Read the model definition and answer for the solid it produces. Units are mm, in the model's axes. A direction names the side the tool comes from. Round coordinates to 2 decimals unless told otherwise and drop trailing zeros. Order: outer loops, then holes, each group sorted by start corner. A loop starts at its lowest first (then second) coordinate and runs counter-clockwise, first axis right, second up. Notation, with made-up numbers: (28.5, 25) - (63.5, 25) arc R21 ccw to (63.5, 55) - close; hole circle Ø11 at (62.5, 3.5). An arc over 180 degrees is marked (long way). One line per question, with ' | ' between items. Start each with the question number.
1) The part is cut by section D-D, the plane x = -1.5. Give the vertices of the cut face in (y, z), plus the area to 3 significant figures.
2) Flat-ended cylindrical pins translate along their axes: pin 1 (2.5 mm diameter, centred on y = -5, z = 0, fed in from +X); pin 2 (0.5 mm diameter, centred on x = 2, y = -3, fed in from -Z); pin 3 (1.5 mm diameter, centred on y = -4, z = 0, fed in from -X). Find the tip coordinate at first contact, or state that the pin passes through.
3) For faces 1 (the flat face through (4.5, -1, 0)), 2 (the flat face through (-1.25, -4, 1)), 3 (the flat face through (2, -3, 3)), 4 (the flat face through (-2, -3, -3)), determine the directions among +Z, -Z, +X, -X, +Y, -Y from which every point of the face is accessible in a straight line to the end or side of a thin tool.
4) Straight lines are drawn through the part: line 1 (Z direction, x = 2, y = -5); line 2 (X direction, y = -4.5, z = 2.5); line 3 (Y direction, x = -3.25, z = 2.75). For each, find the intervals that lie inside material, in ascending order. Write a range as from..to.
5) The part is cut by section C-C, the plane z = 0. Give the vertices of the cut face in (x, y), plus the area to 3 significant figures.
6) The part is cut by section B-B, the plane y = -0.75. Give the vertices of the cut face in (x, z), plus the area to 3 significant figures.
7) The part is cut by section A-A, the plane x = 0. Give the vertices of the cut face in (y, z).
8) The mould has two halves that part along Z. Classify faces 5 (the flat face through (-2, -3, 3)), 6 (the flat face through (2, -3, -3)), 7 (the cylindrical face through (2.1, -5.8, -0.6)), 8 (the flat face through (2, -7, 0)): pulls with the +Z half, pulls with the -Z half, needs draft (parallel to the pull), parting line crosses it, or undercut.
from build123d import *

# Parameters (mm, degrees)
F0_W     = 2.5
F0_H     = 6
F0_R     = 1.2
F1_DEPTH = 2
F0_W_2   = 1.75
F2_DEPTH = 7
F3_R     = 1
F4_DEPTH = 6
F5_R     = 2
F6_R     = 2


with BuildPart() as f1:
    # F0 (on Front) → F1 (new body)
    with BuildSketch(Plane.XZ):
        with BuildLine():
            Line((-3.5, -4.5), (3.5, -4.5))
            ThreePointArc((3.5, -4.5), (4.2071067812, -4.2071067812), (4.5, -3.5))
            Line((4.5, -3.5), (4.5, 3.5))
            ThreePointArc((4.5, 3.5), (4.2071067812, 4.2071067812), (3.5, 4.5))
            Line((3.5, 4.5), (-3.5, 4.5))
            ThreePointArc((-3.5, 4.5), (-4.2071067812, 4.2071067812), (-4.5, 3.5))
            Line((-4.5, 3.5), (-4.5, -3.5))
            ThreePointArc((-4.5, -3.5), (-4.2071067812, -4.2071067812), (-3.5, -4.5))
        make_face()
        Polygon((3, 3), (3, -3), (1.25, -3), (-1.25, -3), (-3, -3), (-3, 3), (-1.25, 3), (1.25, 3), align=None, mode=Mode.SUBTRACT)
        Rectangle(F0_W, F0_H)
        Circle(F0_R, mode=Mode.SUBTRACT)
    extrude(amount=F1_DEPTH)

    # F0 (on Front) → F2 (join)
    with BuildSketch(Plane.XZ):
        with Locations((-2.125, 0)):
            Rectangle(F0_W_2, F0_H)
        with Locations((2.125, 0)):
            Rectangle(F0_W_2, F0_H)
    extrude(amount=F2_DEPTH)

    # F3 (on face) → F4 (cut)
    with BuildSketch(Plane.YZ.offset(3)):
        with Locations((-5, 0)):
            Circle(F3_R)
    extrude(amount=-F4_DEPTH, mode=Mode.SUBTRACT)

    # F5
    f5_edges = [f1.edges().sort_by_distance(p)[0] for p in [
        (2.125, -7, 3),
    ]]
    fillet(f5_edges, radius=F5_R)

    # F6
    f6_edges = [f1.edges().sort_by_distance(p)[0] for p in [
        (-2.125, -7, 3),
        (-2.125, -7, -3),
        (2.125, -7, -3),
    ]]
    fillet(f6_edges, radius=F6_R)


solid = f1.part
Values:
1) outline: (-7, -1) arc R2 ccw to (-5, -3) - (-2, -3) - (-2, -4.5) - (0, -4.5) - (0, 4.5) - (-2, 4.5) - (-2, 3) - (-5, 3) arc R2 ccw to (-7, 1) - close; hole circle Ø2 at (-5, 0) | area: 43.1 mm^2
2) pin 1: stops at x = 3 | pin 2: stops at z = -3 | pin 3: stops at x = -3
3) face 1: +Z, -Z, +X, +Y, -Y | face 2: +Z, -Z, -Y | face 3: +Z, +X, -X, -Y | face 4: -Z, +X, -X, -Y
4) line 1: z = -3..-1, 1..3 | line 2: x = -3..-1.25, 1.25..3 | line 3: y = -2..0
5) outline: (-4.5, -2) - (-3, -2) - (-3, -4) - (-1.25, -4) - (-1.25, -2) - (-1.2, -2) - (-1.2, 0) - (-4.5, 0) - close; (-3, -7) - (-1.25, -7) - (-1.25, -6) - (-3, -6) - close; (1.2, -2) - (1.25, -2) - (1.25, -4) - (3, -4) - (3, -2) - (4.5, -2) - (4.5, 0) - (1.2, 0) - close; (1.25, -7) - (3, -7) - (3, -6) - (1.25, -6) - close | area: 23.7 mm^2
6) outline: (-4.5, -3.5) arc R1 ccw to (-3.5, -4.5) - (3.5, -4.5) arc R1 ccw to (4.5, -3.5) - (4.5, 3.5) arc R1 ccw to (3.5, 4.5) - (-3.5, 4.5) arc R1 ccw to (-4.5, 3.5) - close; hole circle Ø2.4 at (0, 0) | area: 75.6 mm^2
7) outline: (-2, -4.5) - (0, -4.5) - (0, -1.2) - (-2, -1.2) - close; (-2, 1.2) - (0, 1.2) - (0, 4.5) - (-2, 4.5) - close
8) face 5: pulls with the +Z half | face 6: pulls with the -Z half | face 7: undercut | face 8: needs draft
